Design review of the part built by this model. Coordinates are the model's own, in mm. Face numbers are marked on the shaded views. A direction names the side the tool comes from. Coordinates: 2 decimals unless noted, no trailing zeros. Loops run counter-clockwise (first coordinate to the right, second up) from the corner with the lowest first, then second, coordinate; pieces in that order, holes last. Notation, with made-up numbers: M -33.5,83 L 18.5,83 A12 cw 18.5,88 Z; hole C 0.25,7.5 d5. An arc over 180 degrees is marked long. Write item = value, one per line. Start each with the question number.
from build123d import *

# Parameters (mm, degrees)
F0_R        = 47.5
F0_R_2      = 42.5
F1_DEPTH    = 3
F3_DEPTH    = 25
F7_DEPTH    = 5
F8_DEPTH    = 2
F9_T1_DEPTH = 43.7405186698


# Not quite as in the source:
# - a fillet or chamfer that OpenCascade refuses, or shapes differently, is made with other operations: its cross-section is extruded or revolved along the edge and cut away or added


with BuildPart() as f1:
    # F0 (on Top) → F1 (new body)
    with BuildSketch(Plane.XY):
        Circle(F0_R)
        Circle(F0_R_2, mode=Mode.SUBTRACT)
    extrude(amount=F1_DEPTH)

    # F2 (on Top) → F3 (join)
    with BuildSketch(Plane.XY):
        with BuildLine():
            Line((-17.9424604553, 38.4777306174), (-20.0743674327, 43.0496198842))
            ThreePointArc((-20.0743674327, 43.0496198842), (-30.8770370262, 36.0951324209), (-39.4208066889, 26.5))
            Line((-39.4208066889, 26.5), (-33.1695287976, 26.5))
            ThreePointArc((-33.1695287976, 26.5), (-26.2483403101, 33.3690316255), (-17.9424604553, 38.4777306174))
        make_face()
        with BuildLine():
            Line((-20.0743674327, -43.0496198842), (-17.9424604553, -38.4777306174))
            ThreePointArc((-17.9424604553, -38.4777306174), (-26.2483403101, -33.3690316255), (-33.1695287976, -26.5))
            Line((-33.1695287976, -26.5), (-39.4208066889, -26.5))
            ThreePointArc((-39.4208066889, -26.5), (-30.8770370262, -36.0951324209), (-20.0743674327, -43.0496198842))
        make_face()
        with BuildLine():
            Line((20.0743674327, 43.0496198842), (17.9424604553, 38.4777306174))
            ThreePointArc((17.9424604553, 38.4777306174), (26.2483403101, 33.3690316255), (33.1695287976, 26.5))
            Line((33.1695287976, 26.5), (39.4208066889, 26.5))
            ThreePointArc((39.4208066889, 26.5), (30.8770370262, 36.0951324209), (20.0743674327, 43.0496198842))
        make_face()
        with BuildLine():
            ThreePointArc((33.1695287976, -26.5), (26.2483403101, -33.3690316255), (17.9424604553, -38.4777306174))
            Line((17.9424604553, -38.4777306174), (20.0743674327, -43.0496198842))
            ThreePointArc((20.0743674327, -43.0496198842), (30.8770370262, -36.0951324209), (39.4208066889, -26.5))
            Line((39.4208066889, -26.5), (33.1695287976, -26.5))
        make_face()
    extrude(amount=F3_DEPTH)

    # F4 (on face) → F7 (join)
    with BuildSketch(Plane.XY.offset(25)):
        with BuildLine():
            ThreePointArc((39.4208066889, 26.5), (0, 47.5), (-39.4208066889, 26.5))
            Line((-39.4208066889, 26.5), (-33.1695287976, 26.5))
            ThreePointArc((-33.1695287976, 26.5), (0, 42.455478335), (33.1695287976, 26.5))
            Line((33.1695287976, 26.5), (39.4208066889, 26.5))
        make_face()
        with BuildLine():
            Line((-33.1695287976, -26.5), (-39.4208066889, -26.5))
            ThreePointArc((-39.4208066889, -26.5), (0, -47.5), (39.4208066889, -26.5))
            Line((39.4208066889, -26.5), (33.1695287976, -26.5))
            ThreePointArc((33.1695287976, -26.5), (0, -42.455478335), (-33.1695287976, -26.5))
        make_face()
    extrude(amount=F7_DEPTH)

    # F6 (on offset) → F8 (join)
    with BuildSketch(Plane.XY.offset(25)):
        with BuildLine():
            ThreePointArc((-29.4712756106, -30.6217882215), (0, -42.5), (29.4712756106, -30.6217882215))
            Line((29.4712756106, -30.6217882215), (29.4712756106, -23.6217882215))
            ThreePointArc((29.4712756106, -23.6217882215), (0, -37.7696301928), (-29.4712756106, -23.6217882215))
            Line((-29.4712756106, -23.6217882215), (-29.4712756106, -30.6217882215))
        make_face()
        with BuildLine():
            Line((29.4712756106, 23.6217882215), (29.4712756106, 30.6217882215))
            ThreePointArc((29.4712756106, 30.6217882215), (0, 42.5), (-29.4712756106, 30.6217882215))
            Line((-29.4712756106, 30.6217882215), (-29.4712756106, 23.6217882215))
            ThreePointArc((-29.4712756106, 23.6217882215), (0, 37.7696301928), (29.4712756106, 23.6217882215))
        make_face()
    extrude(amount=F8_DEPTH)

    # F9: fillet of radius 4 on 4 edges, made by hand

    # F9_s2 → F9_t1 (cut)
    with BuildSketch(Plane.XY.offset(4.1297406651)):
        with BuildLine():
            ThreePointArc((-29.4712756106, -30.5599665337), (-26.7517914385, -28.7057144703), (-23.5623277872, -29.5188359213))
            ThreePointArc((-23.5623277872, -29.5188359213), (-26.6802279831, -26.7340681466), (-29.4712756106, -23.6217882215))
            Line((-29.4712756106, -23.6217882215), (-29.4712756106, -30.5599665337))
        make_face()
        with BuildLine():
            ThreePointArc((23.5623277872, -29.5188359213), (26.7517914385, -28.7057144703), (29.4712756106, -30.5599665337))
            Line((29.4712756106, -30.5599665337), (29.4712756106, -23.6217882215))
            ThreePointArc((29.4712756106, -23.6217882215), (26.6802279831, -26.7340681466), (23.5623277872, -29.5188359213))
        make_face()
        with BuildLine():
            ThreePointArc((29.4712756106, 30.5599665337), (26.7517914385, 28.7057144703), (23.5623277872, 29.5188359213))
            ThreePointArc((23.5623277872, 29.5188359213), (26.6802279831, 26.7340681466), (29.4712756106, 23.6217882215))
            Line((29.4712756106, 23.6217882215), (29.4712756106, 30.5599665337))
        make_face()
        with BuildLine():
            ThreePointArc((-23.5623277872, 29.5188359213), (-26.7517914385, 28.7057144703), (-29.4712756106, 30.5599665337))
            Line((-29.4712756106, 30.5599665337), (-29.4712756106, 23.6217882215))
            ThreePointArc((-29.4712756106, 23.6217882215), (-26.6802279831, 26.7340681466), (-23.5623277872, 29.5188359213))
        make_face()
    extrude(amount=F9_T1_DEPTH, mode=Mode.SUBTRACT)


solid = f1.part
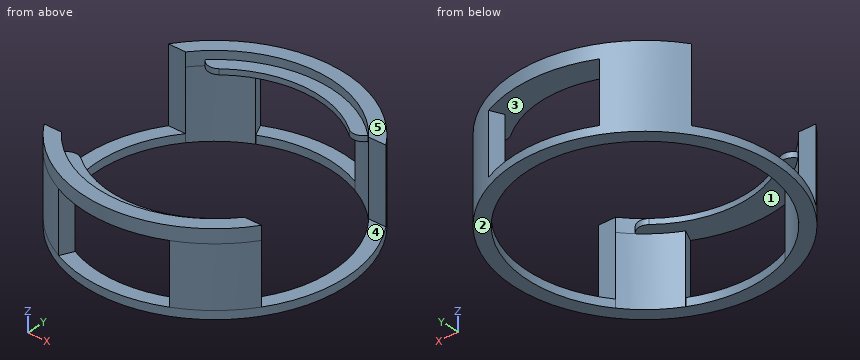
Q1. To check wall thickness, follow line 1 (Y direction, x = 36, z = 28.75); line 2 (Y direction, x = 27, z = 3.25); line 3 (Z direction, x = 8.5, y = -40.5). State the ranges of each line that lie inside material, in increasing order. Write a range as from..to.
Q2. Mouldability with a two-part tool opening along Y and no side actions: class the marked faces 1 and 2 as released by +Y, released by -Y, zero draft, split by the parting line, or undercut.
Q3. Add section B-B on x = 0. State the section outline as (y, z) points.
Q4. Add section A-A on z = 13.25. State the section outline as (x, y) points.
Q5. Add section D-D on x = 11. State the section outline as (y, z) points, plus the area to 3 significant figures.
Q6. Add section C-C on y = 0. State the section outline as (x, z) points, plus the area to 3 significant figures.
Q7. For the marked faces 3, 4 and 5, list the 3-axis set-ups (+Z, -Z, +X, -X, +Y, -Y) from which the entire face can be reached by the end or side of a thin tool; tool diameter is ignored.
Q8. Clearance check with flat-ended pins moving along their axes: P1, Ø1.5, axis at y = 37.5, z = 8.5, coming from the -X side; P2, Ø11.5, axis at x = -42, y = 2.5, coming from the +Z side; P3, Ø10, axis at x = -34.5, z = 21, coming from the -Y side; P4, Ø6, axis at x = 13.5, z = 10.5, coming from the -Y side. State where each tip first meets the part, or that it passes through.
Values follow:
q1.line_1 = -30.99..-26.5, 26.5..30.99
q1.line_2 = -39.08..-32.76, 32.76..39.08
q1.line_3 = 25..27
q2.face_1 = undercut
q2.face_2 = zero draft
q3.outline = M -47.5,0 L -42.5,0 L -42.5,3 L -47.5,3 Z; M -47.5,25 L -37.77,25 L -37.77,27 L -42.46,27 L -42.46,30 L -47.5,30 Z; M 37.77,25 L 47.5,25 L 47.5,30 L 42.46,30 L 42.46,27 L 37.77,27 Z; M 42.5,0 L 47.5,0 L 47.5,3 L 42.5,3 Z
q4.outline = M -39.42,-26.5 A47.5 ccw -20.07,-43.05 L -17.94,-38.48 A42.46 cw -33.17,-26.5 Z; M -39.42,26.5 L -33.17,26.5 A42.46 cw -17.94,38.48 L -20.07,43.05 A47.5 ccw Z; M 17.94,-38.48 L 20.07,-43.05 A47.5 ccw 39.42,-26.5 L 33.17,-26.5 A42.46 cw Z; M 17.94,38.48 A42.46 cw 33.17,26.5 L 39.42,26.5 A47.5 ccw 20.07,43.05 Z
q5.outline = M -46.21,0 L -41.05,0 L -41.05,3 L -46.21,3 Z; M -46.21,25 L -36.13,25 L -36.13,27 L -41.01,27 L -41.01,30 L -46.21,30 Z; M 36.13,25 L 46.21,25 L 46.21,30 L 41.01,30 L 41.01,27 L 36.13,27 Z; M 41.05,0 L 46.21,0 L 46.21,3 L 41.05,3 Z
q5.area = 102 mm2
q6.outline = M -47.5,0 L -42.5,0 L -42.5,3 L -47.5,3 Z; M 42.5,0 L 47.5,0 L 47.5,3 L 42.5,3 Z
q6.area = 30.0 mm2
q7.face_3 = none
q7.face_4 = +Z, +X, -X
q7.face_5 = +Z, +X, -X, +Y, -Y
q8.P1 = -30.09
q8.P2 = 3
q8.P3 = -37.23
q8.P4 = through
